Source: CAD feature listing. Evaluate the final solid. Frame: model axes, mm. A direction names the side the tool comes from. Give positions to 0.01 mm unless a question says otherwise; leave off trailing zeros. Order: outer loops, then holes, each group sorted by start corner. A loop starts at its lowest first (then second) coordinate and runs counter-clockwise, first axis right, second up.
Autodesk Inventor part; units mm, degrees
ref_plane "YZ Plane" through (0, 0, 0) normal (1, 0, 0) x (0, 1, 0)
ref_plane "XZ Plane" through (0, 0, 0) normal (0, 1, 0) x (-1, 0, 0)
ref_plane "XY Plane" through (0, 0, 0) normal (0, 0, 1) x (1, 0, 0)
sketch "Sketch1" plane through (0, 0, 0) normal (0, 0, 1) x (1, 0, 0)
  line L0 (-50, 50) -> (50, 50)
  line L1 (50, 50) -> (50, -50)
  line L2 (50, -50) -> (-50, -50)
  line L3 (-50, -50) -> (-50, 50)
  line L4 (0, 0) -> (0, 10.7298) construction
  line L5 (0, 0) -> (15.4092, 0) construction
  dimension "d0" = 100
  dimension "d1" = 100
extrude "Extrusion1" add sketch "Sketch1" along normal blind 20
sketch "Sketch2" plane through (50, -50, 0) normal (1, 0, 0) x (0, 0, -1)
  line L0 (-20, 100) -> (-20, 0)
  line L1 (-20, 15) -> (-10, 9.2265)
  line L2 (-10, 9.2265) -> (-10, 90.7735)
  line L3 (-10, 90.7735) -> (-20, 85)
  line L4 (0, 0) -> (-20, 0)
  line L5 (0, 100) -> (-20, 100)
  point P0 (0, 50)
  dimension "d4" = 60
  dimension "d5" = 60
  dimension "d6" = 10
  dimension "d9" = 15
  dimension "d10" = 15
extrude "Extrusion2" cut sketch "Sketch2" against normal blind 115.5
sketch "Sketch4" plane through (0, 0, 20) normal (0, 0, 1) x (1, 0, 0)
  line L0 (-50, -50) -> (50, -50)
  line L1 (-50, -35) -> (-50, -50)
  line L2 (50, -50) -> (50, -35)
  line L3 (-50, 50) -> (-50, 35)
  line L4 (50, 50) -> (-50, 50)
  line L5 (50, 35) -> (50, 50)
  circle A0 centre (-40, -45) radius 3
  circle A1 centre (40, -45) radius 3
  circle A2 centre (-40, 45) radius 3
  circle A3 centre (40, 45) radius 3
  point P0 (0, 0)
  dimension "d28" = 5
  dimension "d29" = 10
  dimension "d30" = 5
  dimension "d31" = 10
  dimension "d32" = 10
  dimension "d33" = 5
  dimension "d34" = 10
  dimension "d35" = 5
  dimension "d36" = 6
  dimension "d37" = 6
  dimension "d38" = 6
  dimension "d39" = 6
extrude "Extrusion3" cut sketch "Sketch4" against normal blind 0.3
sketch "Sketch5" plane through (-40, 45, 19.7) normal (0, 0, 1) x (1, 0, 0)
  circle A0 centre (0, -90) radius 3
  circle A1 centre (0, 0) radius 3
  circle A2 centre (80, 0) radius 3
  circle A3 centre (80, -90) radius 3
  point P0 (40, -45)
hole "Hole2" at (-40, -45, 19.7) at (-40, 45, 19.7) at (40, 45, 19.7) at (40, -45, 19.7) direction (0, 0, -1) diameter 2.459 end through all countersink diameter 6 countersink angle 90
sketch "Sketch6" plane through (-50, -50, 0) normal (0, -1, 0) x (1, 0, 0)
  line L0 (0, 20) -> (100, 20)
  line L1 (100, 0) -> (0, 0)
  line L2 (100, 0) -> (100, 20)
  line L3 (0, 0) -> (0, 20)
  point P0 (50, 0)
  point P1 (75, 14)
  point P2 (50, 0)
  point P3 (25, 14)
  dimension "d49" = 6
  dimension "d57" = 25
  dimension "d65" = 25
hole "Hole3" at (25, -50, 14) at (-25, -50, 14) direction (0, 1, 0) diameter 3.242 end through all
sketch "Sketch7" plane through (-50, -50, 0) normal (0, -1, 0) x (1, 0, 0)
  circle A0 centre (14, 5) radius 1.6
  circle A1 centre (5, 5) radius 1.6
  point P0 (50, 0)
hole "Hole4" at (-45, -50, 5) at (-36, -50, 5) direction (0, 1, 0) diameter 2.459 depth 9 tip angle 118
properties part number "3d_LM-Welding_Tooling - Upper fixed base" material "Aluminium 6061-T6"
1) Section query A-A, the plane y = -45. Return the cut outline in (x, z).
Report:
outline: (-50, 0) - (-41.23, 0) - (-41.23, 17.93) - (-43, 19.7) - (-43, 20) - (-50, 20) - close; (-38.77, 0) - (38.77, 0) - (38.77, 17.93) - (37, 19.7) - (37, 20) - (-37, 20) - (-37, 19.7) - (-38.77, 17.93) - close; (41.23, 0) - (50, 0) - (50, 20) - (43, 20) - (43, 19.7) - (41.23, 17.93) - close; hole circle Ø2.46 at (-45, 5); hole circle Ø2.46 at (-36, 5); hole circle Ø3.24 at (-25, 14); hole circle Ø3.24 at (25, 14)
2) Section query C-C, the plane x = -18. Return the cut outline in (y, z), and give its area (3 significant figures).
Report:
outline: (-50, 0) - (50, 0) - (50, 20) - (35, 20) - (40.77, 10) - (-40.77, 10) - (-35, 20) - (-50, 20) - close
area: 1,240 mm2
3) Reachability of faces 4 (the cylindrical face through (-37.22, -45.44, 5.16)), 5 (the cylindrical face through (38.78, -44.84, 8.84)), 6 (the cylindrical face through (41.61, 47.53, 19.85)), 7 (the flat face through (1, -1, 10)) from +Z, -Z, +X, -X, +Y, -Y: full face, straight path, thin tool, end or side. Return the list, or none.
Report:
face 4: -Y
face 5: +Z, -Z
face 6: +Z
face 7: +X, -X
4) Section query B-B, the plane y = 45. Return the cut outline in (x, z), and give its area (3 significant figures).
Report:
outline: (-50, 0) - (-41.23, 0) - (-41.23, 17.93) - (-43, 19.7) - (-43, 20) - (-50, 20) - close; (-38.77, 0) - (38.77, 0) - (38.77, 17.93) - (37, 19.7) - (37, 20) - (-37, 20) - (-37, 19.7) - (-38.77, 17.93) - close; (41.23, 0) - (50, 0) - (50, 20) - (43, 20) - (43, 19.7) - (41.23, 17.93) - close; hole circle Ø3.24 at (-25, 14); hole circle Ø3.24 at (25, 14)
area: 1,880 mm2
5) Section query D-D, the plane y = 8. Return the cut outline in (x, z), and give its area (3 significant figures).
Report:
outline: (-50, 0) - (50, 0) - (50, 10) - (-50, 10) - close
area: 1,000 mm2
6) Draft query along Z for faces 1 (the flat face through (-1, -42, 20)), 2 (the cylindrical face through (-41.22, 45.16, 8.84)), 3 (the cylindrical face through (25.986, 43.845, 15.286)). Return one class per face: +Z half, -Z half, draft (parallel to the pull), parting line (faces both ways), or undercut.
Report:
face 1: +Z half
face 2: draft
face 3: undercut
7) Pin query (flat end, axial travel): pin 1 (10 mm diameter, centred on x = 10, y = -26.5, fed in from -Z); pin 2 (1.5 mm diameter, centred on x = 4.5, y = -17.5, fed in from +Z); pin 3 (3.5 mm diameter, centred on x = -40, y = 45, fed in from +Z); pin 4 (2 mm diameter, centred on x = -45, z = 5, fed in from -Y). Return the tip coordinate at first contact, or that it passes through.
Report:
pin 1: stops at z = 0
pin 2: stops at z = 10
pin 3: stops at z = 18.45
pin 4: stops at y = -40.86
8) Material intervals for L1, parallel to Y at x = -40, z = 19.95; L2, parallel to X at y = 45, z = 19.8; L3, parallel to X at y = -45, z = 7.5, sorted ascending.
Report:
L1: y = -50 to -48, -42 to -35.03, 35.03 to 42, 48 to 50
L2: x = -50 to -43, -37 to 37, 43 to 50
L3: x = -50 to -41.23, -38.77 to 38.77, 41.23 to 50
